The figure shows three views and two pictorial views of one solid part (mm, origin at its lowest corner). Answer the questions. A direction names the side the tool comes from. Coordinates: 2 decimals unless noted, no trailing zeros. Write each loop counter-clockwise with the first axis right and the second up, starting at its lowest first coordinate (ties: lowest second). Pieces come first, ordered by that corner, then holes.
Item 1: Section D-D (y = 9) is taken. Give the vertices of the cut face in (x, z).
Item 2: Each of these flat-tipped pins is pushed along its axis until it touches: P1, Ø4, axis at x = 17.5, z = 8.5, coming from the -Y side; P2, Ø1, axis at x = 7, y = 1.5, coming from the -Z side; P3, Ø1.8, axis at y = 5.5, z = 6, coming from the +X side; P4, Ø4.5, axis at x = 2.5, z = 8.5, coming from the +Y side. Where does it stop, or does it pass through?
Item 3: Section B-B (z = 7.5) is taken. Give the vertices of the cut face in (x, y), then the cut area to 3 significant figures.
Item 4: A tool of negligible diameter and unlimited length cuts with its end or side. For the marked faces 4, 5 and 6, from which of +Z, -Z, +X, -X, +Y, -Y can it reach the whole face along a straight path? Write none if from no direction.
Item 5: Straight lines are drawn through the part: probe 1 along Z at (x, y) = (11, 2); probe 2 along Z at (x, y) = (3, 2.3); probe 3 along Y at (x, z) = (11.25, 3.25). For each, find the intervals that lie inside material, in ascending order.
Item 6: Section A-A (x = 3) is taken. Give the vertices of the cut face in (y, z).
Item 7: Section C-C (x = 11) is taken. Give the vertices of the cut face in (y, z).
Item 8: Determine the mould class of the marked faces 1, 2 and 3 for opening direction Z: released by +Z, released by -Z, zero draft, split by the parting line, or undercut.
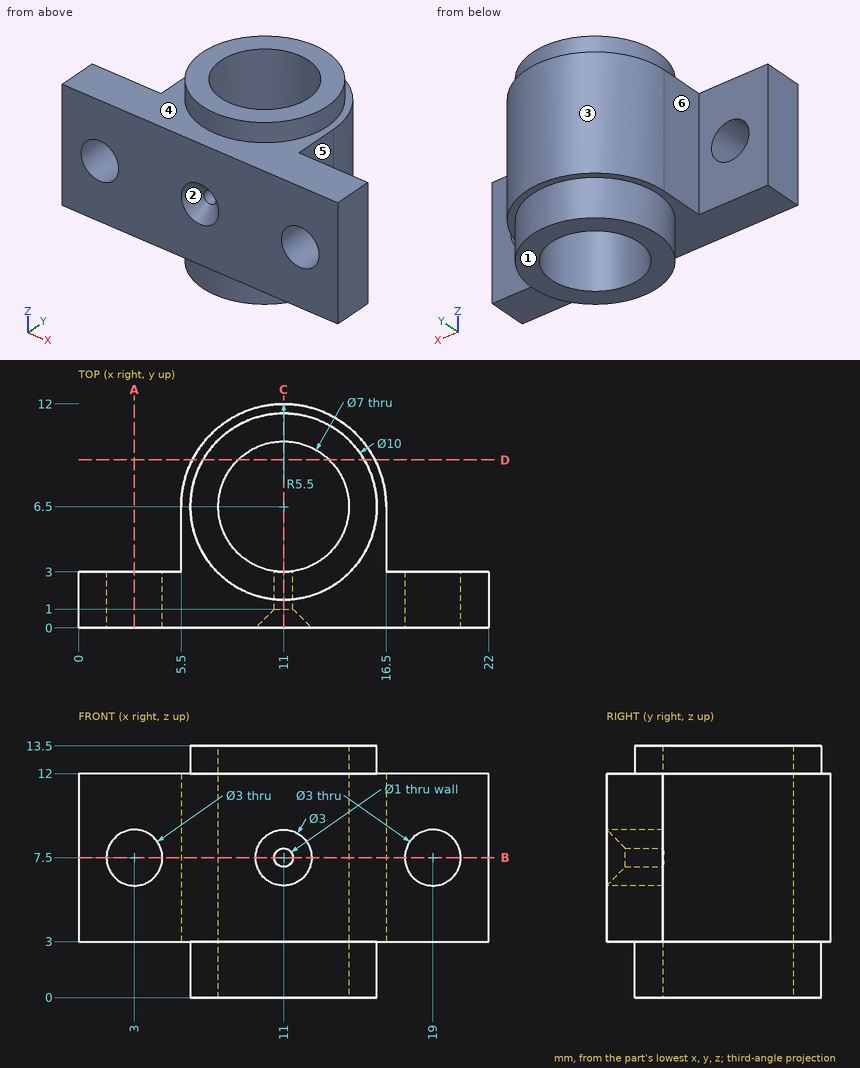
Established:
1. outline: (6.1, 3) - (6.67, 3) - (6.67, 0) - (8.55, 0) - (8.55, 13.5) - (6.67, 13.5) - (6.67, 12) - (6.1, 12) - close; (13.45, 0) - (15.33, 0) - (15.33, 3) - (15.9, 3) - (15.9, 12) - (15.33, 12) - (15.33, 13.5) - (13.45, 13.5) - close
2. P1: stops at y = 0
2. P2: stops at z = 3
2. P3: stops at x = 16.5
2. P4: stops at y = 3
3. outline: (0, 0) - (1.5, 0) - (1.5, 3) - (0, 3) - close; (4.5, 0) - (9.5, 0) - (10.5, 1) - (10.5, 3.04) arc R3.5 cw (long way) to (11.5, 3.04) - (11.5, 1) - (12.5, 0) - (17.5, 0) - (17.5, 3) - (16.5, 3) - (16.5, 6.5) arc R5.5 ccw to (5.5, 6.5) - (5.5, 3) - (4.5, 3) - close; (20.5, 0) - (22, 0) - (22, 3) - (20.5, 3) - close
3. area: 91.5 mm2
4. face 4: +Z
4. face 5: +Z, -Z, +X, +Y
4. face 6: +Z, -Z, -X, +Y
5. probe 1: z = 0 to 7, 8 to 13.5
5. probe 2: z = 3 to 6, 9 to 12
5. probe 3: y = 0 to 3.01, 9.99 to 11.99
6. outline: (0, 3) - (3, 3) - (3, 6) - (0, 6) - close; (0, 9) - (3, 9) - (3, 12) - (0, 12) - close
7. outline: (0, 3) - (1.5, 3) - (1.5, 0) - (3, 0) - (3, 7) - (1, 7) - (0, 6) - close; (0, 9) - (1, 8) - (3, 8) - (3, 13.5) - (1.5, 13.5) - (1.5, 12) - (0, 12) - close; (10, 0) - (11.5, 0) - (11.5, 3) - (12, 3) - (12, 12) - (11.5, 12) - (11.5, 13.5) - (10, 13.5) - close
8. face 1: released by -Z
8. face 2: undercut
8. face 3: zero draft
